Answer from the drawing. Dimensions are ordinates in mm from the lowest x, y and z of the part. Coordinates: 2 decimals unless noted, no trailing zeros. Write each loop counter-clockwise with the first axis right and the second up, starting at its lowest first coordinate (ties: lowest second). Pieces come first, ordered by that corner, then holes. Notation, with made-up numbers: (-21.75, -19) - (-3.75, -19) arc R23 ccw to (-3.75, 15) - close; hole circle Ø10 at (26.25, 55). An arc over 180 degrees is marked (long way). Use one line per item in the form item = value. Start each with the question number.
Item 1: A cutting plane is placed at D-D (z = 41.5). Write down the section's boundary in (x, y), then the cut area to 3 significant figures.
Item 2: Consider probe 1 along X at (y, z) = (2.5, 49.5); probe 2 along Z at (x, y) = (83, 3.5) (1 decimal); probe 3 along Z at (x, y) = (33, 7.75) (1 decimal). Determine where each line is inside the solid, lowest interval first.
Item 3: Determine the mould class of the marked faces 1, 2 and 3 for opening direction Z: released by +Z, released by -Z, zero draft, split by the parting line, or undercut.
Item 4: A cutting plane is placed at B-B (z = 85). Give the number of separate pieces and of enclosed holes in the cut face.
Item 5: A cutting plane is placed at C-C (y = 3.5). Write down the section's boundary in (x, z).
Item 6: A cutting plane is placed at A-A (x = 50). Write down the section's boundary in (y, z), then the cut area to 3 significant figures.
Item 7: Given pin 1 (1.5 mm diameter, centred on y = 4.5, z = 22.5, fed in from -X), flat-ended and moving along its own axis, determine where the tip first touches the part or whether it passes through.
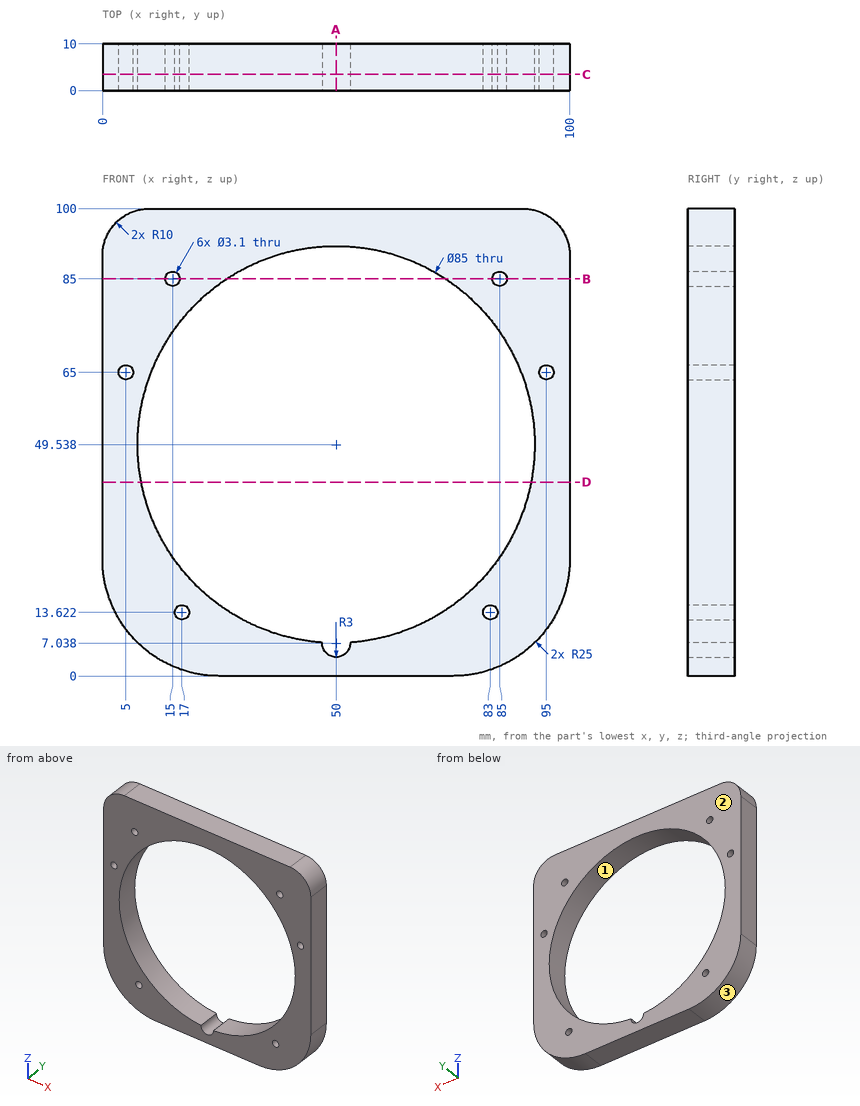
Answer:
q1.outline = (0, 0) - (8.27, 0) - (8.27, 10) - (0, 10) - close; (91.73, 0) - (100, 0) - (100, 10) - (91.73, 10) - close
q1.area = 165 mm²
q2.probe_1 = 0 to 7.5, 92.5 to 100
q2.probe_2 = 1.3 to 12.1, 15.2 to 22.8, 76.3 to 100
q2.probe_3 = 0 to 10.6, 88.5 to 100
q3.face_1 = undercut
q3.face_2 = zero draft
q3.face_3 = released by -Z
q4.separate_pieces = 4
q4.enclosed_holes = 0
q5.outline = (0, 25) arc R25 ccw to (25, 0) - (75, 0) arc R25 ccw to (100, 25) - (100, 90) arc R10 ccw to (90, 100) - (10, 100) arc R10 ccw to (0, 90) - close; hole circle Ø3.1 at (5, 65); hole circle Ø3.1 at (15, 85); hole circle Ø3.1 at (17, 13.62); hole (47, 7.14) arc R3 ccw (long way) to (53, 7.14) arc R42.5 ccw (long way) to start; hole circle Ø3.1 at (83, 13.62); hole circle Ø3.1 at (85, 85); hole circle Ø3.1 at (95, 65)
q6.outline = (0, 0) - (10, 0) - (10, 4.04) - (0, 4.04) - close; (0, 92.04) - (10, 92.04) - (10, 100) - (0, 100) - close
q6.area = 120 mm²
q7.pin_1 = 0.06
